For this review, take the finished solid that the model builds, in its own axes (mm). Round coordinates to 2 decimals unless told otherwise and drop trailing zeros. Loops run counter-clockwise (first coordinate to the right, second up) from the corner with the lowest first, then second, coordinate; pieces in that order, holes last.
1) Wall thickness on L1, parallel to Y at x = 0, z = 2.9; L2, parallel to Y at x = 0, z = 4.8; L3, parallel to Y at x = 27, z = 2.1: over which ranges is each line inside the solid? List them lowest first.
2) Insertion check: pin 1 (2.5 mm diameter, centred on x = -23.38, y = -13.5, fed in from +Z). The pin has a flat end and moves straight along its axis. Give the tip position at first contact, or say it passes through.
3) Take a section at A-A (x = 0). State the section outline as (y, z) points.
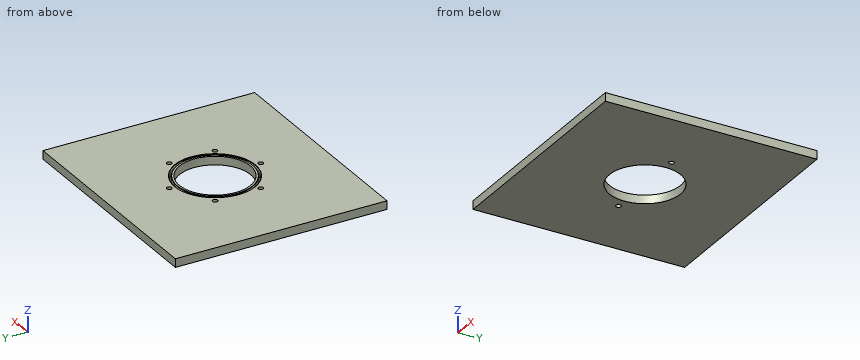
```python
from build123d import *

# Parameters (mm, degrees)
SKETCH1_W           = 135
SKETCH1_H           = 125
SKETCH1_R           = 21
BOSS_EXTRUDE1_DEPTH = 5
CUT_EXTRUDE1_START  = 5
SKETCH1_3_R         = 1.5
CUT_EXTRUDE1_DEPTH  = 3
SKETCH2_R           = 1.5
CUT_EXTRUDE2_DEPTH  = 3


with BuildPart() as part:
    # Sketch1 → Boss-Extrude1 (new body)
    with BuildSketch(Plane.XY):
        Rectangle(SKETCH1_W, SKETCH1_H)
        Circle(SKETCH1_R, mode=Mode.SUBTRACT)
    extrude(amount=BOSS_EXTRUDE1_DEPTH)

    # Sketch1<3> → Cut-Extrude1 (cut)
    with BuildSketch(Plane.XY.offset(CUT_EXTRUDE1_START)):
        with Locations((0, 27)):
            Circle(SKETCH1_3_R)
        with Locations((23.382685902, 13.5)):
            Circle(SKETCH1_3_R)
        with Locations((23.382685902, -13.5)):
            Circle(SKETCH1_3_R)
        with Locations((0, -27)):
            Circle(SKETCH1_3_R)
        with Locations((-23.382685902, -13.5)):
            Circle(SKETCH1_3_R)
        with Locations((-23.382685902, 13.5)):
            Circle(SKETCH1_3_R)
    extrude(amount=-CUT_EXTRUDE1_DEPTH, mode=Mode.SUBTRACT)

    # Sketch2 → Cut-Extrude2 (cut)
    with BuildSketch(Plane(origin=(0, 0, 0), x_dir=(-1, 0, 0), z_dir=(0, 0, -1))):
        with Locations((27, 0)):
            Circle(SKETCH2_R)
        with Locations((-27, 0)):
            Circle(SKETCH2_R)
    extrude(amount=-CUT_EXTRUDE2_DEPTH, mode=Mode.SUBTRACT)

    # Sketch3 → Cut-Revolve1 (revolve, cut)
    with BuildSketch(Plane(origin=(0, 0, 0), x_dir=(0, 0, -1), z_dir=(1, 0, 0))):
        with BuildLine():
            Line((-5, 23.8), (-4.5, 23.8))
            ThreePointArc((-4.5, 23.8), (-4.146446609, 23.653553391), (-4, 23.3))
            Line((-4, 23.3), (-4, 22.7))
            ThreePointArc((-4, 22.7), (-4.146446609, 22.346446609), (-4.5, 22.2))
            Line((-4.5, 22.2), (-5, 22.2))
            Line((-5, 22.2), (-5, 23.8))
        make_face()
    revolve(axis=Axis((0, 0, 0), (0, 0, 1)), mode=Mode.SUBTRACT)


solid = part.part
```
Response:
1. L1: y = -62.5 to -28.5, -25.5 to -21, 21 to 25.5, 28.5 to 62.5
1. L2: y = -62.5 to -28.5, -25.5 to -23.8, -22.2 to -21, 21 to 22.2, 23.8 to 25.5, 28.5 to 62.5
1. L3: y = -62.5 to -1.5, 1.5 to 62.5
2. pin 1: stops at z = 2
3. outline: (-62.5, 0) - (-21, 0) - (-21, 5) - (-22.2, 5) - (-22.2, 4.5) arc R0.5 cw to (-22.7, 4) - (-23.3, 4) arc R0.5 cw to (-23.8, 4.5) - (-23.8, 5) - (-25.5, 5) - (-25.5, 2) - (-28.5, 2) - (-28.5, 5) - (-62.5, 5) - close; (21, 0) - (62.5, 0) - (62.5, 5) - (28.5, 5) - (28.5, 2) - (25.5, 2) - (25.5, 5) - (23.8, 5) - (23.8, 4.5) arc R0.5 cw to (23.3, 4) - (22.7, 4) arc R0.5 cw to (22.2, 4.5) - (22.2, 5) - (21, 5) - close
